Read the model definition and answer for the solid it produces. Units are mm, in the model's axes. Face numbers are marked on the shaded views. A direction names the side the tool comes from. Coordinates: 2 decimals unless noted, no trailing zeros. Order: outer loops, then holes, each group sorted by start corner. A loop starts at its lowest first (then second) coordinate and runs counter-clockwise, first axis right, second up. Notation, with made-up numbers: (-30, 73.25) - (15, 73.25) arc R19 cw to (15, 100.25) - close; hole circle Ø5 at (43.5, 58). An arc over 180 degrees is marked (long way). Write item = value, one per line.
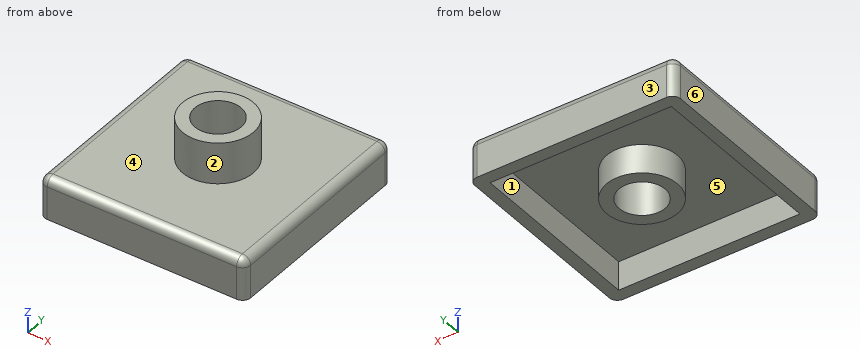
from build123d import *

# Parameters (mm, degrees)
BOSS_EXTRUDE1_DEPTH = 254
SKETCH2_R           = 218.69407086262316
BOSS_EXTRUDE2_DEPTH = 254
FILLET2_R           = 50.8
FILLET3_R           = 50.8
FILLET4_R           = 50.8
FILLET5_R           = 50.8
SKETCH4_R           = 142.49407086262323
CUT_EXTRUDE13_DEPTH = 1867.5111840007871
SHELL4_T            = -76.2


with BuildPart() as part:
    # Sketch1 → Boss-Extrude1 (new body)
    with BuildSketch(Plane.XY):
        Polygon((0, 0), (1270, 0), (1270.0000000000002, -1270), (1.5553e-13, -1270), align=None)
    extrude(amount=BOSS_EXTRUDE1_DEPTH)

    # Sketch2 → Boss-Extrude2 (add)
    with BuildSketch(Plane(origin=(15.756060209551226, -33.262793775725605, 254.0000000000191), x_dir=(1, 0, 0), z_dir=(0, 0, 1))):
        with Locations((633.2493266433831, -595.6098494761216)):
            Circle(SKETCH2_R)
    extrude(amount=BOSS_EXTRUDE2_DEPTH)

    # Fillet2
    fillet2_edges = [part.edges().sort_by_distance(p)[0] for p in [
        (1270, -635, 254),
    ]]
    fillet(fillet2_edges, radius=FILLET2_R)

    # Fillet3
    fillet3_edges = [part.edges().sort_by_distance(p)[0] for p in [
        (609.6, 0, 254),
        (1270, 0, 101.60000000000001),
        (1255.1210244842766, 6.43e-15, 239.12102448427663),
    ]]
    fillet(fillet3_edges, radius=FILLET3_R)

    # Fillet4
    fillet4_edges = [part.edges().sort_by_distance(p)[0] for p in [
        (1270.0000000000002, -1270, 101.60000000000001),
        (1255.1210244842769, -1270, 239.12102448427663),
        (609.6000000000003, -1270, 254),
    ]]
    fillet(fillet4_edges, radius=FILLET4_R)

    # Fillet5
    fillet5_edges = [part.edges().sort_by_distance(p)[0] for p in [
        (0, 0, 101.60000000000001),
        (7.777e-14, -635, 254),
        (6.22e-15, -14.878975515723361, 239.12102448427663),
        (1.5553e-13, -1270, 101.60000000000001),
        (2.2737e-13, -1255.1210244842766, 239.12102448427663),
    ]]
    fillet(fillet5_edges, radius=FILLET5_R)

    # Sketch4 → Cut-Extrude13 (cut, through all)
    with BuildSketch(Plane.XY.offset(508.0000000000191)):
        with Locations((649.0053868529344, -628.8726432518471)):
            Circle(SKETCH4_R)
    extrude(amount=-CUT_EXTRUDE13_DEPTH, mode=Mode.SUBTRACT)

    # Shell4
    shell4_openings = [part.faces().sort_by_distance(p)[0] for p in [
        (635, -1252.039487758, 0),
    ]]
    offset(amount=SHELL4_T, openings=shell4_openings, kind=Kind.INTERSECTION)


solid = part.part
1) The part is cut by section D-D (y = -516). Determine the outline of the cut face in (x, z), and give its area (3 significant figures).
Returned:
outline = (0, 0) - (76.2, 0) - (76.2, 177.8) - (461.69, 177.8) - (461.69, 0) - (562.03, 0) - (562.03, 508) - (461.69, 508) - (461.69, 254) - (50.8, 254) arc R50.8 ccw to (0, 203.2) - close; (735.98, 0) - (836.32, 0) - (836.32, 177.8) - (1193.8, 177.8) - (1193.8, 0) - (1270, 0) - (1270, 203.2) arc R50.8 ccw to (1219.2, 254) - (836.32, 254) - (836.32, 508) - (735.98, 508) - close
area = 196,000 mm^2
2) Flat-ended cylindrical pins translate along their axes: pin 1 Ø8 at (x, z) = (1120, 248) entering from -Y; pin 2 Ø5 at (x, y) = (329.5, -409) entering from -Z; pin 3 Ø2 at (x, y) = (1069, -1001.5) entering from +Z. Find the tip coordinate at first contact, or state that the pin passes through.
Returned:
pin_1 = -1249.47
pin_2 = 177.8
pin_3 = 254
3) Determine the mould class of the marked faces 4, 5 and 6 for opening direction X: pulls with the +X half, pulls with the -X half, needs draft (parallel to the pull), parting line crosses it, or undercut.
Returned:
face_4 = needs draft
face_5 = undercut
face_6 = pulls with the -X half
4) Straight lines are drawn through the part: line 1 along X through (y, z) = (-191.5, 27); line 2 along X through (y, z) = (-815.5, 56); line 3 along Z through (x, y) = (234, -1031). For each, find the intervals that lie inside material, in ascending order. Write a range as from..to.
Returned:
line_1 = 0..76.2, 1193.8..1270
line_2 = 0..76.2, 535..763.01, 1193.8..1270
line_3 = 177.8..254
5) For the marked faces 1, 2 and 3, determine the directions among +Z, -Z, +X, -X, +Y, -Y from which every point of the face is accessible in a straight line to the end or side of a thin tool.
Returned:
face_1 = -Z
face_2 = +Z
face_3 = +Z, -Z, +X, -X, +Y
6) The part is cut by section C-C (y = -1141). Determine the outline of the cut face in (x, z), and give its area (3 significant figures).
Returned:
outline = (0, 0) - (76.2, 0) - (76.2, 177.8) - (1193.8, 177.8) - (1193.8, 0) - (1270, 0) - (1270, 203.2) arc R50.8 ccw to (1219.2, 254) - (50.8, 254) arc R50.8 ccw to (0, 203.2) - close
area = 123,000 mm^2
7) The part is cut by section A-A (z = 139.5). Determine the outline of the cut face in (x, y).
Returned:
outline = (0, -1219.2) arc R50.8 ccw to (50.8, -1270) - (1219.2, -1270) arc R50.8 ccw to (1270, -1219.2) - (1270, -50.8) arc R50.8 ccw to (1219.2, 0) - (50.8, 0) arc R50.8 ccw to (0, -50.8) - close; circle Ø437.39 at (649.01, -628.87); hole (76.2, -1193.8) - (1193.8, -1193.8) - (1193.8, -76.2) - (76.2, -76.2) - close; hole circle Ø284.99 at (649.01, -628.87)
8) The part is cut by section B-B (x = 1168). Determine the outline of the cut face in (y, z), and give its area (3 significant figures).
Returned:
outline = (-1270, 0) - (-1193.8, 0) - (-1193.8, 177.8) - (-76.2, 177.8) - (-76.2, 0) - (0, 0) - (0, 203.2) arc R50.8 ccw to (-50.8, 254) - (-1219.2, 254) arc R50.8 ccw to (-1270, 203.2) - close
area = 123,000 mm^2
